Could you check a few things on this model? Use its own coordinates, in mm. A direction names the side the tool comes from. Give positions to 0.01 mm unless a question says otherwise; leave off trailing zeros. Loops run counter-clockwise (first coordinate to the right, second up) from the corner with the lowest first, then second, coordinate; pieces in that order, holes last. Notation, with made-up numbers: (70.5, 52.5) -> (126.5, 52.5) arc R27 cw to (126.5, 85.5) -> close; hole circle Ø11 at (-32.5, 37.25). An arc over 180 degrees is marked (long way). Put each result on its own line as item: value.
```python
from build123d import *

# Parameters (mm, degrees)
SKETCH1_R                                           = 125
PLATE_DEPTH                                         = 20
CBORE_FOR_M5_HEX_SOCKET_HEAD_CAP_SCREW1_D           = 5.3
CBORE_FOR_M5_HEX_SOCKET_HEAD_CAP_SCREW1_CBORE_D     = 10
CBORE_FOR_M5_HEX_SOCKET_HEAD_CAP_SCREW1_CBORE_DEPTH = 15.4
CIRPATTERN1_COUNT                                   = 3


with BuildPart() as part:
    # Sketch1 → Plate (new body)
    with BuildSketch(Plane(origin=(0, 0, 0), x_dir=(1, 0, 0), z_dir=(0, 1, 0))):
        Circle(SKETCH1_R)
    extrude(amount=PLATE_DEPTH)

    # CBORE for M5 Hex Socket Head Cap Screw1 (through all)
    with Locations(Plane(origin=(0, 20, 0), x_dir=(1, 0, 0), z_dir=(0, 1, 0))):
        with Locations((-105, 0)):
            cbore_for_m5_hex_socket_head_cap_screw1 = CounterBoreHole(CBORE_FOR_M5_HEX_SOCKET_HEAD_CAP_SCREW1_D / 2, CBORE_FOR_M5_HEX_SOCKET_HEAD_CAP_SCREW1_CBORE_D / 2, CBORE_FOR_M5_HEX_SOCKET_HEAD_CAP_SCREW1_CBORE_DEPTH)

    # CirPattern1: CBORE for M5 Hex Socket Head Cap Screw1 ×3 about axis
    cirpattern1_axis = Axis((0, 0, 0), (0, 1, 0))
    for i in range(1, CIRPATTERN1_COUNT):
        add(cbore_for_m5_hex_socket_head_cap_screw1.rotate(cirpattern1_axis, i * 360 / CIRPATTERN1_COUNT), mode=Mode.SUBTRACT)


solid = part.part
```
1. If we section it at C-C (z = -77.5): List the corners of the cut face in (x, y) for me.
Recorded:
outline: (-98.08, 0) -> (98.08, 0) -> (98.08, 20) -> (-98.08, 20) -> close
2. Thinking about a two-plate mould opening in Z: for faces 3 (the face through (-124.88, 9.86, -5.5)), 4 (the face through (-100.381, 12.408, 1.915)), 5 (the face through (-2, 0, -2)), which applies, pulls with the +Z half, pulls with the -Z half, needs draft (parallel to the pull), parting line crosses it, or undercut?
Recorded:
face 3: parting line crosses it
face 4: undercut
face 5: needs draft
3. I need wall thicknesses on line 1 (Z direction, x = 52.5, y = 8); line 2 (Z direction, x = -0.5, y = 16.5); line 3 (Z direction, x = 52.5, y = 3.4). Which ranges of each line are inside material? Lowest first, please.
Recorded:
line 1: z = -113.44 to -95.93, -85.93 to 85.93, 95.93 to 113.44
line 2: z = -125 to 125
line 3: z = -113.44 to -93.58, -88.28 to 88.28, 93.58 to 113.44
4. If we section it at B-B (y = 8.5): List the corners of the cut face in (x, z) for me, then the cut area to 3 significant figures.
Recorded:
outline: circle Ø250 at (0, 0); hole circle Ø10 at (-105, 0); hole circle Ø10 at (52.5, -90.93); hole circle Ø10 at (52.5, 90.93)
area: 48,900 mm^2
5. For faces 1 (the face through (-2, 20, -2)), 2 (the face through (49.6, 4.6, -90.1)), which set-ups out of +Z, -Z, +X, -X, +Y, -Y let a thin tool reach every point of the face, with its end or its side?
Recorded:
face 1: +Z, -Z, +X, -X, +Y
face 2: +Y
6. I'm going to push flat-ended pins straight in: pin 1 (3 mm diameter, centred on x = -104.5, z = 1, fed in from +Y); pin 2 (4 mm diameter, centred on x = 95.5, y = 16, fed in from +Z); pin 3 (8 mm diameter, centred on y = 6.5, z = -28, fed in from -X); pin 4 (3 mm diameter, centred on y = 2, z = -22.5, fed in from -X). Where does each tip first touch, or does it pass through?
Recorded:
pin 1: passes through
pin 2: stops at z = 82.96
pin 3: stops at x = -122.67
pin 4: stops at x = -123.22
7. If we section it at A-A (x = -44): List the corners of the cut face in (y, z) for me, then the cut area to 3 significant figures.
Recorded:
outline: (0, -117) -> (20, -117) -> (20, 117) -> (0, 117) -> close
area: 4,680 mm^2
